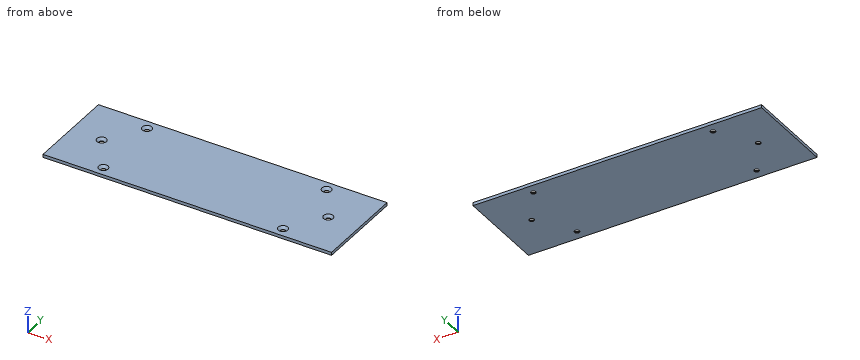
```python
from build123d import *

# Parameters (mm, degrees)
SKETCH1_W                                       = 299.999999694
SKETCH1_H                                       = 93.649999898
BOSS_EXTRUDE1_DEPTH                             = 3.175
CSK_FOR_10_FLAT_HEAD_MACHINE_SCREW1_D           = 5.1054
CSK_FOR_10_FLAT_HEAD_MACHINE_SCREW1_DEPTH       = 4.826
CSK_FOR_10_FLAT_HEAD_MACHINE_SCREW1_CSINK_D     = 9.779
CSK_FOR_10_FLAT_HEAD_MACHINE_SCREW1_CSINK_ANGLE = 82
CSK_FOR_10_FLAT_HEAD_MACHINE_SCREW1_TIP         = 1.533816902
CSK_FOR_10_FLAT_HEAD_MACHINE_SCREW2_D           = 5.1054
CSK_FOR_10_FLAT_HEAD_MACHINE_SCREW2_DEPTH       = 4.826
CSK_FOR_10_FLAT_HEAD_MACHINE_SCREW2_CSINK_D     = 9.779
CSK_FOR_10_FLAT_HEAD_MACHINE_SCREW2_CSINK_ANGLE = 82
CSK_FOR_10_FLAT_HEAD_MACHINE_SCREW2_TIP         = 1.533816902


with BuildPart() as part:
    # Sketch1 → Boss-Extrude1 (new body)
    with BuildSketch(Plane.XY):
        Rectangle(SKETCH1_W, SKETCH1_H)
    extrude(amount=BOSS_EXTRUDE1_DEPTH)

    # CSK for #10 Flat Head Machine Screw1
    with Locations(Plane.XY.offset(3.175)):
        with Locations((-93.374999847, 36.824999949), (93.374999847, 36.824999949), (93.374999847, -36.824999949), (-93.374999847, -36.824999949)):
            CounterSinkHole(CSK_FOR_10_FLAT_HEAD_MACHINE_SCREW1_D / 2, CSK_FOR_10_FLAT_HEAD_MACHINE_SCREW1_CSINK_D / 2, depth=CSK_FOR_10_FLAT_HEAD_MACHINE_SCREW1_DEPTH, counter_sink_angle=CSK_FOR_10_FLAT_HEAD_MACHINE_SCREW1_CSINK_ANGLE)
            with Locations((0, 0, -(CSK_FOR_10_FLAT_HEAD_MACHINE_SCREW1_DEPTH + CSK_FOR_10_FLAT_HEAD_MACHINE_SCREW1_TIP / 2))):  # 118° drill point
                Cone(0, CSK_FOR_10_FLAT_HEAD_MACHINE_SCREW1_D / 2, CSK_FOR_10_FLAT_HEAD_MACHINE_SCREW1_TIP, mode=Mode.SUBTRACT)

    # CSK for #10 Flat Head Machine Screw2
    with Locations(Plane.XY.offset(3.175)):
        with Locations((-117.774999847, 0), (117.774999847, 0)):
            CounterSinkHole(CSK_FOR_10_FLAT_HEAD_MACHINE_SCREW2_D / 2, CSK_FOR_10_FLAT_HEAD_MACHINE_SCREW2_CSINK_D / 2, depth=CSK_FOR_10_FLAT_HEAD_MACHINE_SCREW2_DEPTH, counter_sink_angle=CSK_FOR_10_FLAT_HEAD_MACHINE_SCREW2_CSINK_ANGLE)
            with Locations((0, 0, -(CSK_FOR_10_FLAT_HEAD_MACHINE_SCREW2_DEPTH + CSK_FOR_10_FLAT_HEAD_MACHINE_SCREW2_TIP / 2))):  # 118° drill point
                Cone(0, CSK_FOR_10_FLAT_HEAD_MACHINE_SCREW2_D / 2, CSK_FOR_10_FLAT_HEAD_MACHINE_SCREW2_TIP, mode=Mode.SUBTRACT)


solid = part.part
```
Input: part model. Units: mm. Frame: model coordinates. Coordinates: 2 decimals unless noted, no trailing zeros. Loops run counter-clockwise (first coordinate to the right, second up) from the corner with the lowest first, then second, coordinate; pieces in that order, holes last. Notation, with made-up numbers: (-5, 9) -> (33, 9) arc R37 cw to (33, 46) -> close; hole circle Ø9 at (30.5, -21.5). An arc over 180 degrees is marked (long way). Use a Markdown table: item, result.
1) Contact query for flat-ended pins moving along their axis: pin 1 (8 mm diameter, centred on x = -35.5, y = 24.5, fed in from -Z); pin 2 (8 mm diameter, centred on x = -93.375, y = 36.825, fed in from +Z). Output: stop coordinate, or through.
Results found:
| item | result |
|---|---|
| pin 1 | stops at z = 0 |
| pin 2 | stops at z = 2.15 |
2) Cut plane A-A (y = 0). Return the cut outline in (x, z) (1 decimal).
Results found:
| item | result |
|---|---|
| outline | (-150, 0) -> (-120.3, 0) -> (-120.3, 0.5) -> (-122.7, 3.2) -> (-150, 3.2) -> close; (-115.2, 0) -> (115.2, 0) -> (115.2, 0.5) -> (112.9, 3.2) -> (-112.9, 3.2) -> (-115.2, 0.5) -> close; (120.3, 0) -> (150, 0) -> (150, 3.2) -> (122.7, 3.2) -> (120.3, 0.5) -> close |
3) Material intervals for line 1 along X through (y, z) = (-1, 0.6); line 2 along Z through (x, y) = (-115, 3), sorted ascending. Write a range as from..to.
Results found:
| item | result |
|---|---|
| line 1 | x = -150..-120.23, -115.32..115.32, 120.23..150 |
| line 2 | z = 0..2.25 |
